Part print with two shaded views. Sizes in mm from the minimum x, y, z corner. A direction names the side the tool comes from. Round coordinates to 2 decimals unless told otherwise and drop trailing zeros. Order: outer loops, then holes, each group sorted by start corner. A loop starts at its lowest first (then second) coordinate and runs counter-clockwise, first axis right, second up. Notation, with made-up numbers: (13, 1) -> (63, 1) arc R21 cw to (63, 30) -> close; hole circle Ø3 at (66.25, 62). An arc over 180 degrees is marked (long way). Answer as a JSON object with one key per item and string values.
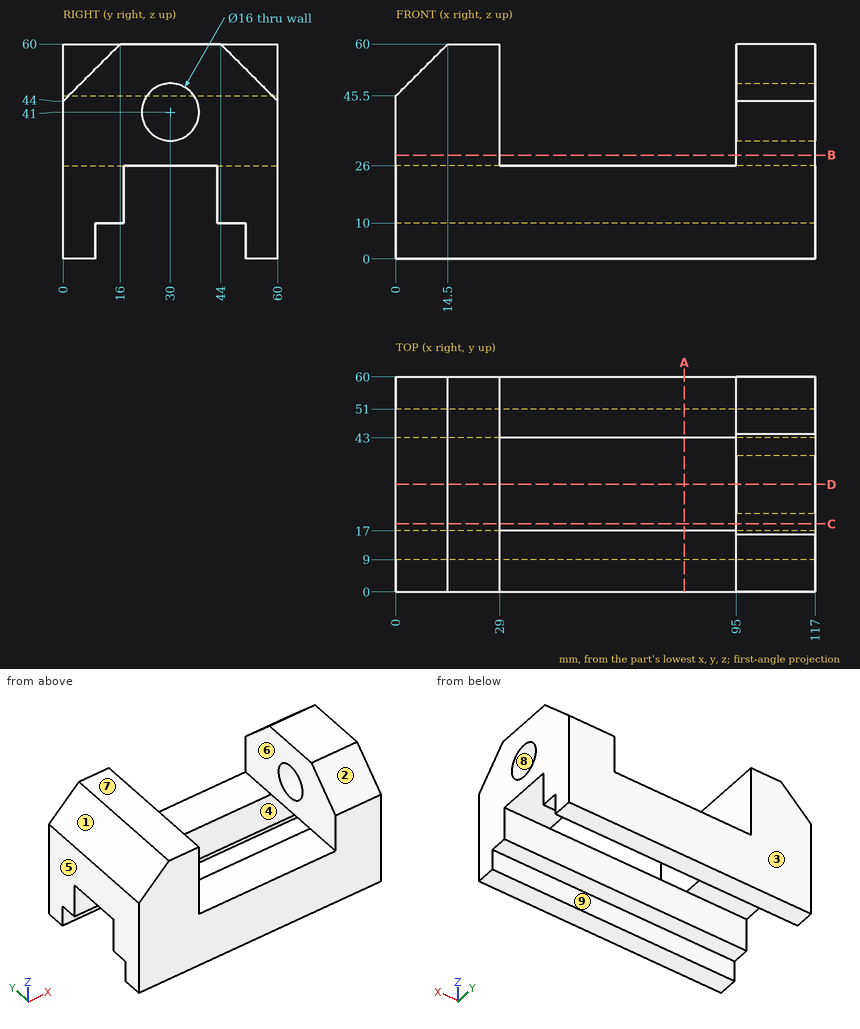
1) Flat gauge pins, fed straight in: pin 1 Ø1.5 at (x, y) = (63, 7) entering from +Z; pin 2 Ø11 at (x, y) = (103, 33.5) entering from -Z; pin 3 Ø6.5 at (x, y) = (48.5, 13) entering from -Z. Where does each tip first touch, or does it go through?
Checked values:
{"pin 1": "stops at z = 26", "pin 2": "stops at z = 26", "pin 3": "stops at z = 10"}
2) Pull direction Y, two halves, no side cores. Call the marked faces 1, 2, 3 and 4: pulls with the +Y half, pulls with the -Y half, needs draft (parallel to the pull), parting line crosses it, or undercut.
Checked values:
{"face 1": "needs draft", "face 2": "pulls with the -Y half", "face 3": "pulls with the +Y half", "face 4": "undercut"}
3) Probe L1, parallel to Z at x = 104, y = 30; L2, parallel to X at y = 50.5, z = 39; L3, parallel to Y at x = 91.5, z = 25.5. List the from-to ranges inside material, lowest first. Write a range as from..to.
Checked values:
{"L1": "z = 26..33, 49..60", "L2": "x = 0..29, 95..117", "L3": "y = 0..17, 43..60"}
4) Cut at C-C, the plane y = 19. Give the cut face in (x, z), plus the area to 3 significant figures.
Checked values:
{"outline": "(0, 26) -> (29, 26) -> (29, 60) -> (14.5, 60) -> (0, 45.5) -> close; (95, 26) -> (117, 26) -> (117, 60) -> (95, 60) -> close", "area": "1,630 mm²"}
5) Cut at B-B, the plane z = 29. Give the cut face in (x, y), plus the area to 3 significant figures.
Checked values:
{"outline": "(0, 0) -> (29, 0) -> (29, 60) -> (0, 60) -> close; (95, 0) -> (117, 0) -> (117, 60) -> (95, 60) -> close", "area": "3,060 mm²"}
6) Cut at D-D, the plane y = 30. Give the cut face in (x, z).
Checked values:
{"outline": "(0, 26) -> (29, 26) -> (29, 60) -> (14.5, 60) -> (0, 45.5) -> close; (95, 26) -> (117, 26) -> (117, 33) -> (95, 33) -> close; (95, 49) -> (117, 49) -> (117, 60) -> (95, 60) -> close"}
7) Which spindle directions (+Z, -Z, +X, -X, +Y, -Y) get a long thin tool onto all of the face, cutting with end or side? Do the marked faces 5, 6, 7, 8 and 9. Say none if no direction does.
Checked values:
{"face 5": "+Z, -Z, -X, +Y, -Y", "face 6": "+Z, +Y, -Y", "face 7": "+Z, +X, -X, +Y, -Y", "face 8": "+X", "face 9": "-Z, +X, -X"}
8) Cut at A-A, the plane x = 80.5. Give the cut face in (y, z).
Checked values:
{"outline": "(0, 0) -> (9, 0) -> (9, 10) -> (17, 10) -> (17, 26) -> (0, 26) -> close; (43, 10) -> (51, 10) -> (51, 0) -> (60, 0) -> (60, 26) -> (43, 26) -> close"}
